For this review, take the finished solid that the model builds, in its own axes (mm). A direction names the side the tool comes from. Coordinates: 2 decimals unless noted, no trailing zeros. Write each loop counter-clockwise with the first axis right and the second up, starting at its lowest first coordinate (ties: lowest second). Pieces come first, ordered by that corner, then holes. Notation, with made-up numbers: (20, 70) - (78, 70) arc R26 ccw to (78, 85) - close; hole circle Ø5 at (20, 2.25). An arc over 180 degrees is marked (long way). Write each question's results on one line, items separated by ' | '.
Autodesk Inventor part; units mm, degrees
ref_plane "YZ Plane" through (0, 0, 0) normal (1, 0, 0) x (0, 1, 0)
ref_plane "XZ Plane" through (0, 0, 0) normal (0, 1, 0) x (-1, 0, 0)
ref_plane "XY Plane" through (0, 0, 0) normal (0, 0, 1) x (1, 0, 0)
sketch "Schizzo1" plane through (0, 0, 0) normal (0, 0, 1) x (1, 0, 0)
  circle A0 centre (0, 0) radius 5
  dimension "d0" = 10
extrude "Estrusione1" add sketch "Schizzo1" along normal blind 15
sketch "Schizzo2" plane through (0, 0, 15) normal (0, 0, 1) x (1, 0, 0)
  circle A0 centre (0, 0) radius 4
  dimension "d3" = 8
extrude "Estrusione2" add sketch "Schizzo2" along normal blind 10
thread "Filettatura1"
chamfer "Smusso1" distance 0.5 angle 45 2 edges at (-4, 0, 25) (-5, 0, 0)
properties part number "Perno tendi motore" material "Acciaio inossidabile"
Q1. For pin 1 (5 mm diameter, centred on y = 3, z = 15.5, fed in from -X); pin 2 (1 mm diameter, centred on x = 1.5, z = 7, fed in from +Y), all flat-tipped, find the tip position at first contact; note any pin that passes through.
Results found:
pin 1: x = -4.97 | pin 2: y = 4.9
Q2. Wall thickness on line 1 along Z through (x, y) = (3, 3); line 2 along Y through (x, z) = (3, 3.75); line 3 along Z through (x, y) = (3.5, 3.25): over which ranges is each line inside the solid? List them lowest first. Write a range as from..to.
Results found:
line 1: 0..15 | line 2: -4..4 | line 3: 0.28..15
Q3. Take a section at A-A on x = 0. State the section outline as (y, z) points.
Results found:
outline: (-5, 0.5) - (-4.5, 0) - (4.5, 0) - (5, 0.5) - (5, 15) - (4, 15) - (4, 24.5) - (3.5, 25) - (-3.5, 25) - (-4, 24.5) - (-4, 15) - (-5, 15) - close
Q4. For faces 1 (the face through (0, 0, 0)), 2 (the face through (-0.867, 3.905, 19.684)), list the 3-axis set-ups (+Z, -Z, +X, -X, +Y, -Y) from which the entire face can be reached by the end or side of a thin tool; tool diameter is ignored.
Results found:
face 1: -Z, +X, -X, +Y, -Y | face 2: +Z
Q5. Take a section at C-C on z = 22.5. State the section outline as (x, y) points, plus the area to 3 significant figures.
Results found:
outline: circle Ø8 at (0, 0) | area: 50.3 mm2
